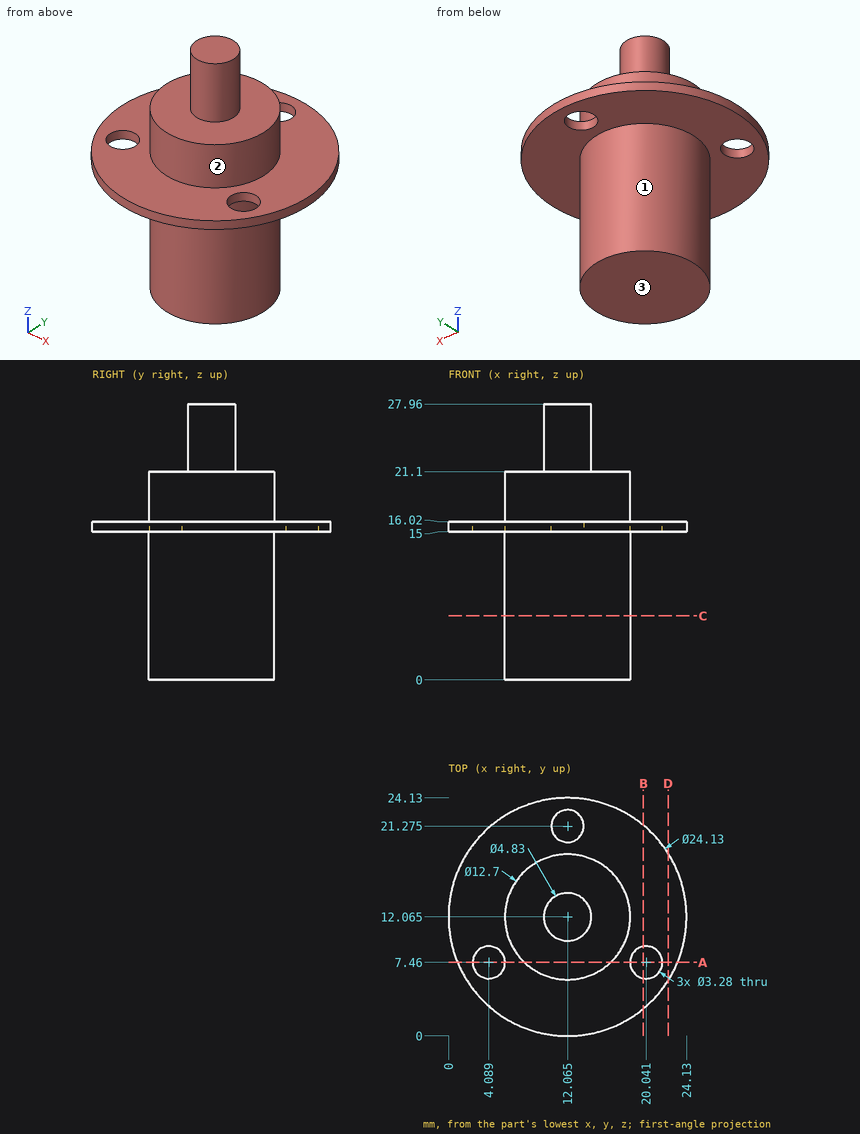
Job drawing, mm, ordinate dimensions from the low corner. One solid piece. A direction names the side the tool comes from. Give positions to 0.01 mm unless a question says otherwise; leave off trailing zeros. Loops run counter-clockwise (first coordinate to the right, second up) from the corner with the lowest first, then second, coordinate; pieces in that order, holes last. Notation, with made-up numbers: (84.25, 44) -> (129.25, 44) arc R27 ccw to (129.25, 73) -> close; hole circle Ø6 at (45.5, 57.5). An arc over 180 degrees is marked (long way). Write each question's results on one line, items separated by ' | '. Start each with the question number.
Q1. Which spindle directions (+Z, -Z, +X, -X, +Y, -Y) get a long thin tool onto all of the face, cutting with end or side? Do the marked faces 1, 2 and 3. Say none if no direction does.
Q2. Pin check, flat tips, straight feed: P1, Ø1, axis at y = 19, z = 18, coming from the +X side; P2, Ø4, axis at y = 18, z = 17, coming from the +X side; P3, Ø1.5, axis at y = 6, z = 10.5, coming from the -X side; P4, Ø10, axis at y = 5.5, z = 18.5, coming from the +X side. Stop position of each tip, or through.
Q3. Band-saw the part on A-A on y = 7.46. List the corners of the cut face in (x, z), plus the area to 3 significant figures.
Q4. Wall check: L1, parallel to Z at x = 18.5, y = 19.5; L2, parallel to Z at x = 6, y = 10.5; L3, parallel to Y at x = 9, z = 18.5. Give the ranges that are in metal, low to high.
Q5. Band-saw the part on B-B on x = 19.75. List the corners of the cut face in (y, z).
Q6. Band-saw the part on D-D on x = 22.25. List the corners of the cut face in (y, z), plus the area to 3 significant figures.
Q7. Band-saw the part on C-C on z = 6.5. List the corners of the cut face in (x, y) (3 decimals), plus the area to 3 significant figures.
Results are:
1) face 1: -Z | face 2: +Z | face 3: -Z, +X, -X, +Y, -Y
2) P1: passes through | P2: stops at x = 23.38 | P3: stops at x = 8.59 | P4: stops at x = 23.92
3) outline: (0.91, 15) -> (2.45, 15) -> (2.45, 16.02) -> (0.91, 16.02) -> close; (5.73, 15) -> (7.69, 15) -> (7.69, 0) -> (16.44, 0) -> (16.44, 15) -> (18.4, 15) -> (18.4, 16.02) -> (16.44, 16.02) -> (16.44, 21.1) -> (7.69, 21.1) -> (7.69, 16.02) -> (5.73, 16.02) -> close; (21.68, 15) -> (23.22, 15) -> (23.22, 16.02) -> (21.68, 16.02) -> close | area: 192 mm²
4) L1: z = 15 to 16.02 | L2: z = 0 to 21.1 | L3: y = 6.5 to 17.63
5) outline: (2.76, 15) -> (5.85, 15) -> (5.85, 16.02) -> (2.76, 16.02) -> close; (9.07, 15) -> (21.37, 15) -> (21.37, 16.02) -> (9.07, 16.02) -> close
6) outline: (5.6, 15) -> (18.53, 15) -> (18.53, 16.02) -> (5.6, 16.02) -> close | area: 13.2 mm²
7) outline: circle Ø12.7 at (12.065, 12.065) | area: 127 mm²
